Here's the drawing with two shaded views (mm, measured from the low corner). I have some questions. A direction names the side the tool comes from. Round coordinates to 2 decimals unless told otherwise and drop trailing zeros. Order: outer loops, then holes, each group sorted by start corner. A loop starts at its lowest first (then second) coordinate and runs counter-clockwise, first axis right, second up.
Q1. We'd pull the mould along X, two halves only. Please class the marked faces 1, 2 and 3: pulls with the +X half, pulls with the -X half, needs draft (parallel to the pull), parting line crosses it, or undercut.
Q2. If we section it at A-A (y = 24.5): Please give me the cut outline in (x, z).
Q3. If I drill on line 1 (Z direction, x = 15.5, y = 13.75); line 2 (X direction, y = 8.5, z = 22.5); line 3 (Y direction, x = 20.25, z = 10), over which ranges is the centre line in solid material (lowest first)?
Q4. If we section it at B-B (z = 18.5): Please give me the cut outline in (x, y), plus the area to 3 significant figures.
Q5. For the marked faces 4, 5, 6 and 7, which set-ups out of +Z, -Z, +X, -X, +Y, -Y let a thin tool reach every point of the face, with its end or its side?
Q6. If we section it at C-C (z = 12): Please give me the cut outline in (x, y).
Q7. Will these pins go through, and if not, where does the flat tip stop? P1, Ø9, axis at x = 28, z = 20, coming from the +Y side; P2, Ø2, axis at x = 14.5, y = 20.5, coming from the -Z side; P3, Ø3, axis at y = 26, z = 7, coming from the +X side; P4, Ø3.5, axis at x = 20.25, y = 24.5, coming from the -Z side.
Q8. If we section it at D-D (y = 4.5): Please give me the cut outline in (x, z).
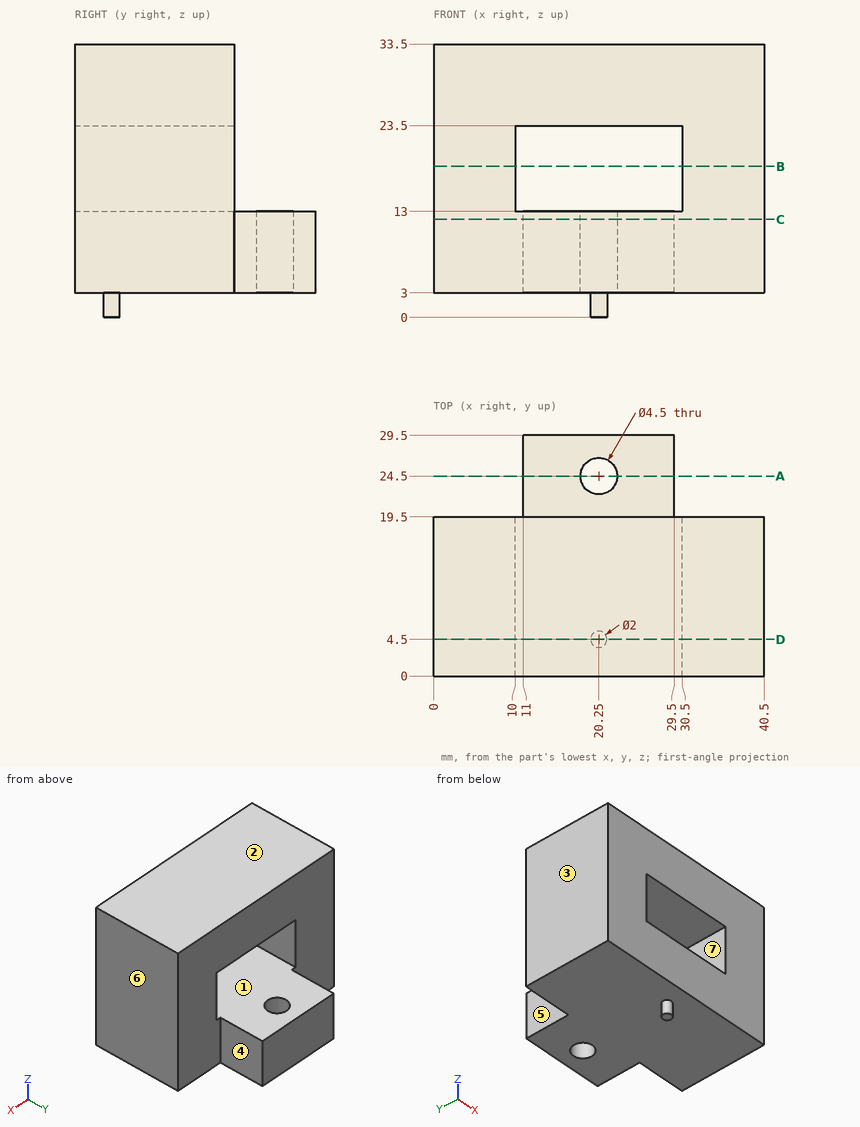
Solution:
1. face 1: undercut
1. face 2: needs draft
1. face 3: pulls with the -X half
2. outline: (11, 3) - (18, 3) - (18, 13) - (11, 13) - close; (22.5, 3) - (29.5, 3) - (29.5, 13) - (22.5, 13) - close
3. line 1: z = 3 to 13, 23.5 to 33.5
3. line 2: x = 0 to 10, 30.5 to 40.5
3. line 3: y = 0 to 22.25, 26.75 to 29.5
4. outline: (0, 0) - (10, 0) - (10, 19.5) - (0, 19.5) - close; (30.5, 0) - (40.5, 0) - (40.5, 19.5) - (30.5, 19.5) - close
4. area: 390 mm2
5. face 4: +Z, -Z, +X, +Y
5. face 5: +Z, -Z, -X, +Y
5. face 6: +Z, -Z, +X, +Y, -Y
5. face 7: +Y, -Y
6. outline: (0, 0) - (40.5, 0) - (40.5, 19.5) - (29.5, 19.5) - (29.5, 29.5) - (11, 29.5) - (11, 19.5) - (0, 19.5) - close; hole circle Ø4.5 at (20.25, 24.5)
7. P1: stops at y = 19.5
7. P2: stops at z = 3
7. P3: stops at x = 29.5
7. P4: passes through
8. outline: (0, 3) - (19.25, 3) - (19.25, 0) - (21.25, 0) - (21.25, 3) - (40.5, 3) - (40.5, 33.5) - (0, 33.5) - close; hole (10, 13) - (30.5, 13) - (30.5, 23.5) - (10, 23.5) - close
